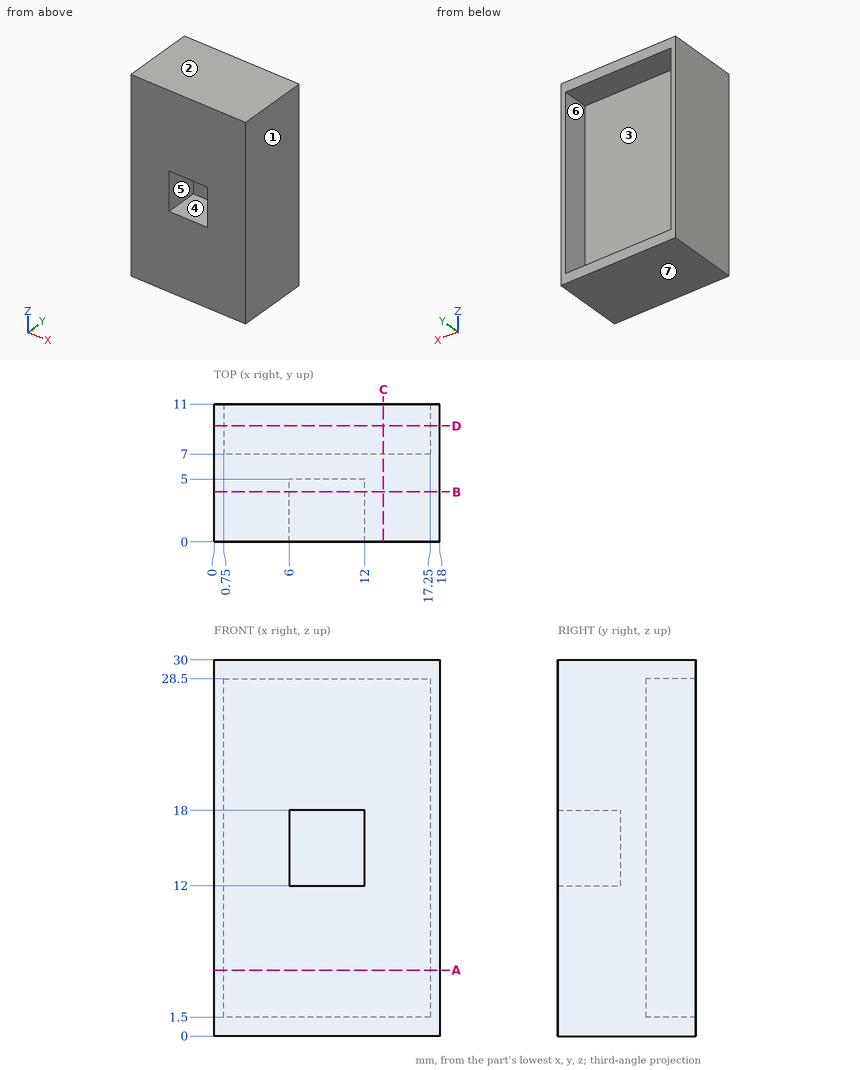
Study the drawing (mm; zero at the part's minimum x, y, z) and answer. A direction names the side the tool comes from. Round coordinates to 2 decimals unless told otherwise and drop trailing zeros. Loops run counter-clockwise (first coordinate to the right, second up) from the corner with the lowest first, then second, coordinate; pieces in that order, holes last. Notation, with made-up numbers: (63.5, 13.5) -> (73.5, 13.5) arc R30 cw to (73.5, 45.5) -> close; hole circle Ø1 at (55.5, 22.25). An arc over 180 degrees is marked (long way). One line per item, written item: value.
1) A cutting plane is placed at A-A (z = 5.25). Determine the outline of the cut face in (x, y), and give its area (3 significant figures).
Answer list:
outline: (0, 0) -> (18, 0) -> (18, 11) -> (17.25, 11) -> (17.25, 7) -> (0.75, 7) -> (0.75, 11) -> (0, 11) -> close
area: 132 mm²
2) Flat-ended cylindrical pins translate along their axes: P1, Ø10, axis at x = 8, z = 21, coming from the +Y side; P2, Ø1, axis at x = 13, z = 18.5, coming from the -Y side; P3, Ø3, axis at x = 9, z = 15.5, coming from the -Y side. Find the tip coordinate at first contact, or state that the pin passes through.
Answer list:
P1: stops at y = 7
P2: stops at y = 0
P3: stops at y = 5
3) A cutting plane is placed at B-B (y = 4). Determine the outline of the cut face in (x, z).
Answer list:
outline: (0, 0) -> (18, 0) -> (18, 30) -> (0, 30) -> close; hole (6, 12) -> (12, 12) -> (12, 18) -> (6, 18) -> close
4) For the marked faces 5, 6 and 7, determine the directions among +Z, -Z, +X, -X, +Y, -Y from which every point of the face is accessible in a straight line to the end or side of a thin tool.
Answer list:
face 5: -Y
face 6: +Y
face 7: -Z, +X, -X, +Y, -Y
5) A cutting plane is placed at D-D (y = 9.25). Determine the outline of the cut face in (x, z).
Answer list:
outline: (0, 0) -> (18, 0) -> (18, 30) -> (0, 30) -> close; hole (0.75, 1.5) -> (17.25, 1.5) -> (17.25, 28.5) -> (0.75, 28.5) -> close
6) A cutting plane is placed at C-C (x = 13.5). Determine the outline of the cut face in (y, z), and give its area (3 significant figures).
Answer list:
outline: (0, 0) -> (11, 0) -> (11, 1.5) -> (7, 1.5) -> (7, 28.5) -> (11, 28.5) -> (11, 30) -> (0, 30) -> close
area: 222 mm²
7) Consider L1, parallel to Z at x = 7, y = 2.75; L2, parallel to X at y = 3, z = 15.75; L3, parallel to Z at x = 5.75, y = 9.25. Determine where each line is inside the solid, lowest interval first. Write a range as [from, to].
Answer list:
L1: z = [0, 12], [18, 30]
L2: x = [0, 6], [12, 18]
L3: z = [0, 1.5], [28.5, 30]
8) The mould has two halves that part along X. Classify the marked faces 1, 2, 3 and 4: pulls with the +X half, pulls with the -X half, needs draft (parallel to the pull), parting line crosses it, or undercut.
Answer list:
face 1: pulls with the +X half
face 2: needs draft
face 3: undercut
face 4: undercut
